Autodesk Inventor part; units mm, degrees
ref_plane "YZ Plane" through (0, 0, 0) normal (1, 0, 0) x (0, 1, 0)
ref_plane "XZ Plane" through (0, 0, 0) normal (0, 1, 0) x (-1, 0, 0)
ref_plane "XY Plane" through (0, 0, 0) normal (0, 0, 1) x (1, 0, 0)
sketch "Sketch1" plane through (0, 0, 0) normal (1, 0, 0) x (0, 1, 0)
  line L0 (-6, -12.5) -> (-6, -12.9)
  arc A0 (-6, -12.9) -> (-5.6, -13.3) centre (-5.6, -12.9) ccw
  line L1 (-5.6, -13.3) -> (-4.9, -13.3)
  arc A1 (-4.9, -13.3) -> (-4.7, -13.1) centre (-4.9, -13.1) ccw
  line L2 (-4.7, -13.1) -> (-4.7, -12.85)
  arc A2 (-4.5, -12.65) -> (-4.7, -12.85) centre (-4.5, -12.85) ccw
  line L3 (-4.5, -12.65) -> (-1.8, -12.65)
  arc A3 (-1.4, -13.05) -> (-1.8, -12.65) centre (-1.8, -13.05) ccw
  line L4 (-1.4, -13.05) -> (-1.4, -18.75)
  line L5 (-1.8, -19.15) -> (-4.5, -19.15)
  arc A4 (-1.8, -19.15) -> (-1.4, -18.75) centre (-1.8, -18.75) ccw
  arc A5 (-4.7, -18.95) -> (-4.5, -19.15) centre (-4.5, -18.95) ccw
  line L6 (-4.7, -18.95) -> (-4.7, -18.7)
  arc A6 (-4.7, -18.7) -> (-4.9, -18.5) centre (-4.9, -18.7) ccw
  line L7 (-4.9, -18.5) -> (-5.6, -18.5)
  arc A7 (-5.6, -18.5) -> (-6, -18.9) centre (-5.6, -18.9) ccw
  line L8 (-6, -18.9) -> (-6, -19.5)
  line L9 (-6.5, -6.5) -> (-6.5, -12.5)
  line L10 (-6.5, -12.5) -> (-2.5, -12.5)
  line L11 (-1.05, -19.5) -> (-6.5, -19.5)
  line L12 (-6.5, -19.5) -> (-6.5, -26)
  line L13 (-6.5, -26) -> (-1.05, -26)
  line L14 (-6, -26) -> (-6, -26.6)
  arc A8 (-6, -26.6) -> (-5.6, -27) centre (-5.6, -26.6) ccw
  line L15 (-5.6, -27) -> (-4.9, -27)
  arc A9 (-4.9, -27) -> (-4.7, -26.8) centre (-4.9, -26.8) ccw
  arc A10 (-4.5, -26.35) -> (-4.7, -26.55) centre (-4.5, -26.55) ccw
  line L16 (-4.7, -26.8) -> (-4.7, -26.55)
  line L17 (-4.5, -26.35) -> (-1.8, -26.35)
  arc A11 (-1.4, -26.75) -> (-1.8, -26.35) centre (-1.8, -26.75) ccw
  line L18 (-1.4, -26.75) -> (-1.4, -32.45)
  arc A12 (-1.8, -32.85) -> (-1.4, -32.45) centre (-1.8, -32.45) ccw
  line L19 (-1.8, -32.85) -> (-4.5, -32.85)
  arc A13 (-4.7, -32.65) -> (-4.5, -32.85) centre (-4.5, -32.65) ccw
  line L20 (-4.7, -32.65) -> (-4.7, -32.4)
  arc A14 (-4.7, -32.4) -> (-4.9, -32.2) centre (-4.9, -32.4) ccw
  line L21 (-4.9, -32.2) -> (-5.6, -32.2)
  arc A15 (-5.6, -32.2) -> (-6, -32.6) centre (-5.6, -32.6) ccw
  line L22 (-6, -32.6) -> (-6, -33)
  line L23 (-2.5, -33) -> (-6.5, -33)
  line L24 (-6.5, -33) -> (-6.5, -39)
  line L25 (32.5, 0) -> (0, 0)
  circle A16 centre (0, -6.5) radius 4.75
  circle A17 centre (32.5, -6.5) radius 4.75
  circle A18 centre (0, -39) radius 4.75
  circle A19 centre (32.5, -39) radius 4.75
  line L26 (39, -26) -> (39, -19.5)
  line L27 (39, -12.5) -> (39, -6.5)
  line L28 (39, -39) -> (39, -33)
  line L29 (26.5, -45.5) -> (32.5, -45.5)
  line L30 (0, -45.5) -> (6, -45.5)
  line L31 (13, -45.5) -> (19.5, -45.5)
  circle A20 centre (16.25, -22.75) radius 15
  circle A21 centre (16.2588, 5.0016) radius 2.5
  circle A22 centre (16.25, -50.5) radius 2.5
  circle A23 centre (16.25, -22.75) radius 5
  circle A24 centre (16.25, -22.75) radius 8.45
  line L32 (24.75, -27.6575) -> (24.75, -17.8425)
  line L33 (44, 10) -> (-11.5, 10)
  line L34 (-11.5, 10) -> (-11.5, -55.5)
  line L35 (-11.5, -55.5) -> (44, -55.5)
  line L36 (44, -55.5) -> (44, 10)
  line L37 (-11.5, 30) -> (44, 30)
  line L38 (-11.5, -75.5) -> (-11.5, 30)
  line L39 (44, 30) -> (44, -75.5)
  line L40 (44, -75.5) -> (-11.5, -75.5)
  circle A25 centre (16.25, -65.5) radius 5
  circle A26 centre (16.25, 20) radius 5
  arc A27 (11.25, -55.5) -> (21.25, -55.5) centre (16.25, -55.5) ccw
  line L41 (21.25, 10) -> (21.25, -55.5)
  line L42 (11.25, -55.5) -> (11.25, 10)
  arc A28 (21.25, 10) -> (11.25, 10) centre (16.25, 10) ccw
  line L43 (21.25, -45.5) -> (11.25, -45.5)
  point P0 (21.25, 0)
  point P1 (11.25, 0)
extrude "Extrusion1" add sketch "Sketch1" along normal blind 10 contours L41 A20 L42 L25 | L41 A24 L42 A20 | L41 A23 L42 A24 | L42 A24 L41 A20 | A20 L41 L43 L31 L42 | A23 | L41 A24 L42 A23
extrude "Extrusion2" add sketch "Sketch1" along normal blind 5 contours L25 L42 L33 L41 | L43 L31 L41 L35 L42
sketch "Sketch2" plane through (10, 11.25, 0) normal (0, 0, 1) x (1, 0, 0)
  line L0 (0, 10) -> (0, 0)
  circle A0 centre (0, 5) radius 7.5
  line L1 (0, 5) -> (11.155, 5)
  line L2 (-5, 10) -> (0, 10)
  line L3 (0, 10) -> (7.5, 5)
  line L4 (7.5, 5) -> (0, 0)
  line L5 (0, 10) -> (7.5, 10)
  line L6 (7.5, 10) -> (0, 5)
  line L7 (0, 5) -> (7.5, 0)
  line L8 (7.5, 0) -> (0, 0)
  point P0 (-10, -11.25)
  point P1 (3.75, 2.5)
  point P2 (3.75, 7.5)
  dimension "d4" = 15
extrude "Extrusion4" add sketch "Sketch2" against normal up to surface (45.5 mm away) contours L3 L6 L0 | L5 A0 L6 L3 | L7 L4 L0 | L5 L6 A0 | L4 L7 A0 L8 | A0 L7 L8
sketch "Sketch3" plane through (0, 11.25, -55.5) normal (0, -1, 0) x (1, 0, 0)
  line L0 (17.5, 55.5) -> (17.5, 10)
  circle A0 centre (17.5, 32.75) radius 2.5
  point P0 (0, 55.5)
  dimension "d9" = 5
extrude "Extrusion5" cut sketch "Sketch3" against normal through all
sketch "Sketch4" plane through (5, 11.25, 0) normal (0, 0, 1) x (1, 0, 0)
  line L0 (12.5, 10) -> (10, 8.3333)
  line L1 (12.5, 10) -> (12.5, 0)
  line L2 (12.5, 0) -> (5, 5)
  line L3 (5, 5) -> (12.5, 10)
  point P0 (-5, -11.25)
extrude "Extrusion6" add sketch "Sketch4" against normal up to surface (45.5 mm away)
sketch "Sketch5" plane through (0, 11.25, -55.5) normal (0, -1, 0) x (1, 0, 0)
  line L0 (17.5, 35.25) -> (17.5, 30.25)
  circle A0 centre (17.5, 32.75) radius 2.5
  point P0 (0, 55.5)
extrude "Extrusion7" cut sketch "Sketch5" against normal through all
properties part number "SoporteTubosInferior_CPY"
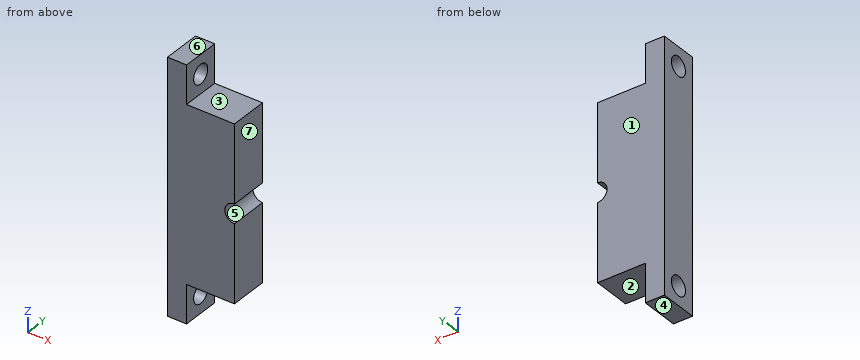
Here's how the part is built. I have some questions about the finished solid (model axes, mm). Face numbers are marked on the shaded views. A direction names the side the tool comes from. Round coordinates to 2 decimals unless told otherwise and drop trailing zeros. Write each loop counter-clockwise with the first axis right and the second up, starting at its lowest first coordinate (ties: lowest second). Pieces come first, ordered by that corner, then holes.
Q1. If we section it at D-D on y = 18: Write out the boundary of the cut face in (x, z).
Q2. If we section it at A-A on z = -50.5: Write out the boundary of the cut face in (x, y).
Q3. Which directions (+Z, -Z, +X, -X, +Y, -Y) give clear straight access to the entire face, cutting with the end or side of a thin tool? Please do the marked faces 1, 2 and 3.
Q4. If we mould it in two halves opening along Z, with no side actions, what happens to the marked faces 4, 5, 6 and 7? For each: +Z half, -Z half, draft (parallel to the pull), parting line (faces both ways), or undercut.
Q5. Please list where these lines run through material, in increasing order: probe 1 along Z at (x, y) = (2.75, 16.25); probe 2 along Z at (x, y) = (2.75, 15.75); probe 3 along X at (y, z) = (19.5, -51).
Q6. Will these pins go through, and if not, where does the flat tip stop? P1, Ø1.5, axis at x = 6, y = 20, coming from the -Z side; P2, Ø5, axis at y = 16.5, z = 7, coming from the +X side; P3, Ø3, axis at x = 12.5, y = 15.5, coming from the +Z side.
Q7. If we section it at B-B on y = 13: Write out the boundary of the cut face in (x, z), plus the area to 3 significant figures.
Q8. If we section it at C-C on x = 1: Write out the boundary of the cut face in (y, z), plus the area to 3 significant figures.
Answer below:
1. outline: (0, -55.5) - (5, -55.5) - (5, -52.29) - (0, -52.29) - close; (0, -48.71) - (5, -48.71) - (5, -45.5) - (17.5, -45.5) - (17.5, -25.25) arc R2.5 cw to (17.5, -20.25) - (17.5, 0) - (5, 0) - (5, 3.21) - (0, 3.21) - close; (0, 6.8) - (5, 6.8) - (5, 10) - (0, 10) - close
2. outline: (0, 11.25) - (5, 11.25) - (5, 13.75) - (0, 13.75) - close; (0, 18.75) - (5, 18.75) - (5, 21.25) - (0, 21.25) - close
3. face 1: +Z, -Z, +X, -X, +Y
3. face 2: -Z, +X, +Y, -Y
3. face 3: +Z, +X, +Y, -Y
4. face 4: -Z half
4. face 5: undercut
4. face 6: +Z half
4. face 7: draft
5. probe 1: z = -55.5 to -53, -48 to 2.5, 7.5 to 10
5. probe 2: z = -55.5 to -52.95, -48.05 to 2.55, 7.45 to 10
5. probe 3: x = 0 to 5
6. P1: stops at z = -45.5
6. P2: stops at x = 5
6. P3: stops at z = 0
7. outline: (0, -55.5) - (5, -55.5) - (5, -45.5) - (17.5, -45.5) - (17.5, -25.25) arc R2.5 cw to (17.5, -20.25) - (17.5, 0) - (5, 0) - (5, 10) - (0, 10) - close
7. area: 886 mm2
8. outline: (11.25, -55.5) - (21.25, -55.5) - (21.25, 10) - (11.25, 10) - close; hole circle Ø5 at (16.25, -50.5); hole circle Ø5 at (16.26, 5)
8. area: 616 mm2
